CAD build for the part. Positions are in the model's coordinates, mm. Coordinates: 2 decimals unless noted, no trailing zeros. Order: outer loops, then holes, each group sorted by start corner. A loop starts at its lowest first (then second) coordinate and runs counter-clockwise, first axis right, second up. Notation, with made-up numbers: M -4,28 L 30,28 A8 ccw 30,40 Z; hole C 76,-31.5 d10. An arc over 180 degrees is marked long. Write item = value, one per line.
from build123d import *

# Parameters (mm, degrees)
SKETCH1_W           = 146
SKETCH1_H           = 161
BOSS_EXTRUDE1_DEPTH = 3
SKETCH2_W           = 26
SKETCH2_H           = 3
SKETCH2_W_2         = 3
SKETCH2_H_2         = 30
SKETCH2_W_3         = 60
SKETCH2_H_3         = 25
CUT_EXTRUDE1_DEPTH  = 3
SKETCH4_R           = 1.7
SKETCH4_R_2         = 6.2
SKETCH4_W           = 98
SKETCH4_H           = 41
CUT_EXTRUDE2_DEPTH  = 3


with BuildPart() as part:
    # Sketch1 → Boss-Extrude1 (new body)
    with BuildSketch(Plane(origin=(0, 0, 0), x_dir=(1, 0, 0), z_dir=(0, 1, 0))):
        Rectangle(SKETCH1_W, SKETCH1_H)
    extrude(amount=BOSS_EXTRUDE1_DEPTH)

    # Sketch2 → Cut-Extrude1 (cut)
    with BuildSketch(Plane(origin=(0, 3, 0), x_dir=(1, 0, 0), z_dir=(0, 1, 0))):
        with Locations((0, 79)):
            Rectangle(SKETCH2_W, SKETCH2_H)
        with Locations((-71.5, 25.5)):
            Rectangle(SKETCH2_W_2, SKETCH2_H_2)
        Polygon((-73, 80.5), (-73, 60.5), (-70, 60.5), (-70, 77.5), (-43, 77.5), (-43, 80.5), align=None)
        Polygon((73, 80.5), (73, 60.5), (70, 60.5), (70, 77.5), (43, 77.5), (43, 80.5), align=None)
        with Locations((71.5, 25.5)):
            Rectangle(SKETCH2_W_2, SKETCH2_H_2)
        with Locations((-71.5, -24.5)):
            Rectangle(SKETCH2_W_2, SKETCH2_H_2)
        Polygon((-70, -59.5), (-73, -59.5), (-73, -80.5), (-43, -80.5), (-43, -77.5), (-70, -77.5), align=None)
        with Locations((71.5, -24.5)):
            Rectangle(SKETCH2_W_2, SKETCH2_H_2)
        Polygon((70, -59.5), (73, -59.5), (73, -80.5), (70, -80.5), (43, -80.5), (43, -77.5), (70, -77.5), align=None)
        with Locations((0, -79)):
            Rectangle(SKETCH2_W, SKETCH2_H)
        with Locations((17, 60)):
            Rectangle(SKETCH2_W_3, SKETCH2_H_3)
    extrude(amount=-CUT_EXTRUDE1_DEPTH, mode=Mode.SUBTRACT)

    # Sketch4 → Cut-Extrude2 (cut)
    with BuildSketch(Plane(origin=(0, 3, 0), x_dir=(1, 0, 0), z_dir=(0, 1, 0))):
        with Locations(Location((-46.5, 35.5, 0), (0, 0, 270))):
            Circle(SKETCH4_R)
        with Locations(Location((46.5, 35.5, 0), (0, 0, 270))):
            Circle(SKETCH4_R)
        with Locations(Location((46.5, -19.5, 0), (0, 0, 270))):
            Circle(SKETCH4_R)
        with Locations(Location((-46.5, -19.5, 0), (0, 0, 270))):
            Circle(SKETCH4_R)
        with Locations(Location((-30.75, -42.3, 0), (0, 0, 270))):
            Circle(SKETCH4_R)
        with Locations(Location((-30.75, -68.5, 0), (0, 0, 270))):
            Circle(SKETCH4_R)
        with Locations(Location((30.75, -42.3, 0), (0, 0, 270))):
            Circle(SKETCH4_R)
        with Locations(Location((30.75, -68.5, 0), (0, 0, 270))):
            Circle(SKETCH4_R)
        with Locations(Location((-10.75, -47.9, 0), (0, 0, 270))):
            Circle(SKETCH4_R_2)
        with Locations(Location((-24, -55.4, 0), (0, 0, 270))):
            Circle(SKETCH4_R_2)
        with Locations(Location((-10.75, -62.9, 0), (0, 0, 270))):
            Circle(SKETCH4_R_2)
        with Locations(Location((2.5, -55.4, 0), (0, 0, 270))):
            Circle(SKETCH4_R_2)
        with Locations(Location((24, -55.4, 0), (0, 0, 270))):
            Circle(SKETCH4_R_2)
        with Locations((0, 8)):
            Rectangle(SKETCH4_W, SKETCH4_H)
    extrude(amount=-CUT_EXTRUDE2_DEPTH, mode=Mode.SUBTRACT)


solid = part.part
(1) Pin check, flat tips, straight feed: pin 1 Ø1 at (x, y) = (-49, 1) entering from +Z; pin 2 Ø0.9 at (x, y) = (62.5, 1.5) entering from -Z; pin 3 Ø0.9 at (x, y) = (71, 1.5) entering from +Z. Stop position of each tip, or through.
Evaluation:
pin_1 = 77.5
pin_2 = -77.5
pin_3 = 59.5
(2) Pull direction Z, two halves, no side cores. Call faces 1 (the face through (25.9, 1.5, 61.3)), 2 (the face through (30.8, 1.5, 66.8)), 3 (the face through (-1, 3, 17)): +Z half, -Z half, draft (parallel to the pull), parting line (faces both ways), or undercut.
Evaluation:
face_1 = undercut
face_2 = undercut
face_3 = draft
(3) Slice it at D-D, the plane z = 24. Write the cut outline in (x, y), then the cut area to 3 significant figures.
Evaluation:
outline = M -70,0 L 70,0 L 70,3 L -70,3 Z
area = 420 mm²
(4) Slice it at A-A, the plane x = -24. Write the cut outline in (y, z), then the cut area to 3 significant figures.
Evaluation:
outline = M 0,-80.5 L 3,-80.5 L 3,-28.5 L 0,-28.5 Z; M 0,12.5 L 3,12.5 L 3,49.2 L 0,49.2 Z; M 0,61.6 L 3,61.6 L 3,80.5 L 0,80.5 Z
area = 323 mm²
(5) Slice it at C-C, the plane y = 2.5. State how many separate pieces and enclosed holes the cut face has, then the cut area to 3 significant figures.
Evaluation:
separate_pieces = 1
enclosed_holes = 15
area = 16,200 mm²
(6) Wall check: line 1 (Z direction, x = 44, y = 2); line 2 (X direction, y = 2.3, z = 55.4); line 3 (Z direction, x = 16.5, y = 1.9). Give the ranges that are in metal, low to high. Write a range as from..to.
Evaluation:
line_1 = -77.5..-72.5, -47.5..-28.5, 12.5..77.5
line_2 = -73..-30.2, -17.8..-3.7, 8.7..17.8, 30.2..73
line_3 = -80.5..-72.5, -47.5..-28.5, 12.5..80.5
(7) Slice it at B-B, the plane x = 24. Write the cut outline in (y, z).
Evaluation:
outline = M 0,-80.5 L 3,-80.5 L 3,-72.5 L 0,-72.5 Z; M 0,-47.5 L 3,-47.5 L 3,-28.5 L 0,-28.5 Z; M 0,12.5 L 3,12.5 L 3,49.2 L 0,49.2 Z; M 0,61.6 L 3,61.6 L 3,80.5 L 0,80.5 Z
